For this review, take the finished solid that the model builds, in its own axes (mm). Face numbers are marked on the shaded views. A direction names the side the tool comes from. Coordinates: 2 decimals unless noted, no trailing zeros. Write each loop counter-clockwise with the first axis right and the second up, starting at its lowest first coordinate (ties: lowest second). Pieces come first, ordered by that corner, then holes. Notation, with made-up numbers: (-5, 50) -> (42, 50) arc R25 ccw to (42, 74) -> close; hole circle Ø8 at (-6.5, -5). An arc over 180 degrees is marked (long way). Put each result on its own line as item: value. Start each with the question number.
Item 1: To check wall thickness, follow L1, parallel to Z at x = -6.5, y = 19.5; L2, parallel to Z at x = 1.5, y = 15; L3, parallel to X at y = 19.25, z = -19.5. State the ranges of each line that lie inside material, in increasing order.
Item 2: Consider section A-A on y = 22. Give the number of separate pieces and of enclosed holes in the cut face, and give its area (3 significant figures).
Item 3: Consider section D-D on x = 8.5. Give the boundary of the cut face in (y, z).
Item 4: Consider section C-C on z = 9. Give the boundary of the cut face in (x, y), and give its area (3 significant figures).
Item 5: Consider section B-B on x = -12. Give the boundary of the cut face in (y, z).
Item 6: Insertion check: P1, Ø8, axis at y = 16.5, z = 10.5, coming from the -X side; P2, Ø4, axis at x = 20, y = 17, coming from the +Z side; P3, Ø1.5, axis at x = 18.5, z = 9, coming from the +Y side. Each pin has a flat end and moves straight along its axis. Give the tip position at first contact, or say it passes through.
Item 7: For the marked faces 1, 2 and 3, list the 3-axis set-ups (+Z, -Z, +X, -X, +Y, -Y) from which the entire face can be reached by the end or side of a thin tool; tool diameter is ignored.
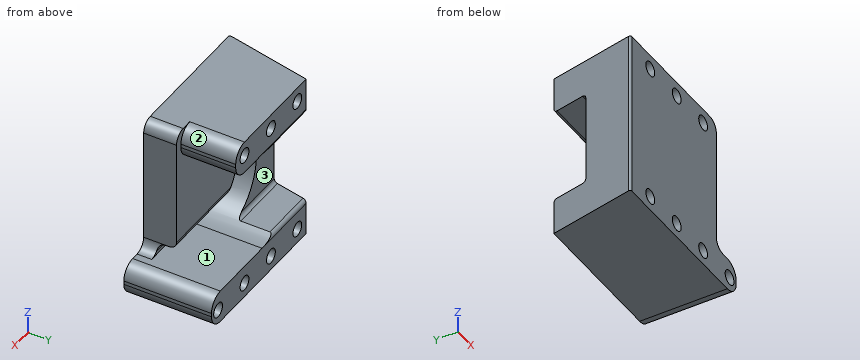
```python
from build123d import *

# Parameters (mm, degrees)
SKETCH2_R           = 2
SKETCH2_R_2         = 2.0000000000000004
SKETCH2_R_3         = 2.0000000000000036
BOSS_EXTRUDE1_DEPTH = 24
BOSS_EXTRUDE2_DEPTH = 46
CUT_EXTRUDE1_START  = -10
CUT_EXTRUDE1_DEPTH  = 10
FILLET1_R           = 1
FILLET2_R           = 0.5
FILLET3_R           = 4
BOSS_EXTRUDE3_START = -9
BOSS_EXTRUDE3_DEPTH = 9
FILLET4_R           = 3
CUT_EXTRUDE2_START  = -5
CUT_EXTRUDE2_DEPTH  = 5
FILLET5_R           = 2


with BuildPart() as part:
    # Sketch2 → Boss-Extrude1 (new body)
    with BuildSketch(Plane(origin=(0, 0, 0), x_dir=(1, 0, 0), z_dir=(0, 1, 0))):
        with BuildLine():
            ThreePointArc((-10.00000000000001, 1.71e-15), (-7.224972160321737, 8.36660026534089), (3.0642e-13, 13.41640786499884))
            ThreePointArc((3.0642e-13, 13.41640786499884), (1.9788258499060016, 13.85333371629342), (4.000000000000001, 14.00000000000001))
            Line((4, 14.00000000000001), (27, 14))
            Line((27, 14), (27, 23.000000000000007))
            Line((27, 23.000000000000007), (-16, 23))
            Line((-16, 23.000000000000004), (-16, -22.999999999999996))
            Line((-16, -22.999999999999996), (15.999999999999996, -22.999999999999993))
            Line((15.999999999999996, -22.999999999999993), (15.999999999999996, -14))
            Line((15.999999999999996, -14), (4, -14.00000000000001))
            ThreePointArc((3.9999999999999973, -14.00000000000001), (-5.899494936611674, -9.899494936611672), (-10.00000000000001, 1.71e-15))
        make_face()
        with Locations(Location((-11.999999999999995, -19, 0), (0, 0, 270))):
            Circle(SKETCH2_R, mode=Mode.SUBTRACT)
        with Locations(Location((4.65e-15, -19, 0), (0, 0, 270))):
            Circle(SKETCH2_R_2, mode=Mode.SUBTRACT)
        with Locations(Location((11.999999999999995, -19, 0), (0, 0, 270))):
            Circle(SKETCH2_R, mode=Mode.SUBTRACT)
        with Locations(Location((-12, 19, 0), (0, 0, 270))):
            Circle(SKETCH2_R_2, mode=Mode.SUBTRACT)
        with Locations(Location((4.7e-16, 19, 0), (0, 0, 270))):
            Circle(SKETCH2_R, mode=Mode.SUBTRACT)
        with Locations(Location((12, 19, 0), (0, 0, 270))):
            Circle(SKETCH2_R, mode=Mode.SUBTRACT)
        with Locations(Location((24.003693078979538, 19, 0), (0, 0, 270))):
            Circle(SKETCH2_R_3, mode=Mode.SUBTRACT)
    extrude(amount=BOSS_EXTRUDE1_DEPTH)

    # Sketch4 → Boss-Extrude2 (add)
    with BuildSketch(Plane.XY.offset(22.999999999999993)):
        Polygon((-21.000000000000004, -1.04e-15), (-16.000000000000004, 24), (-16.000000000000004, 0), align=None)
    extrude(amount=-BOSS_EXTRUDE2_DEPTH)

    # Sketch5 → Cut-Extrude1 (cut)
    with BuildSketch(Plane(origin=(0, 24, 0), x_dir=(1, 0, 0), z_dir=(0, 1, 0)).offset(CUT_EXTRUDE1_START)):
        with BuildLine():
            Line((-16, 0), (-10.000000000000007, 0))
            ThreePointArc((-10.000000000000007, 3.5391e-13), (-7.591939740998584, 7.850282354225094), (-1.1961524227063602, 13.000000000000117))
            Line((-1.196152422706339, 13), (-16, 12.999999999999998))
            Line((-16, 13.000000000000004), (-16, 0))
        make_face()
        Polygon((-21.000000000000004, 0), (-16, 0), (-16, 13.000000000000004), (-21.000000000000004, 12.999999999999998), align=None)
        with BuildLine():
            ThreePointArc((-1.1961524227063673, -13.000000000000114), (-7.591939740998785, -7.850282354224801), (-10.000000000000007, 3.5391e-13))
            Line((-10.000000000000007, 0), (-16, 0))
            Line((-16, 0), (-16, -13))
            Line((-15.999999999999998, -13.000000000000002), (-1.1961524227063371, -13))
        make_face()
        Polygon((-16, -13), (-16, 0), (-21.000000000000004, 0), (-21, -13), align=None)
    extrude(amount=CUT_EXTRUDE1_DEPTH, mode=Mode.SUBTRACT)

    # Fillet1
    fillet1_edges = [part.edges().sort_by_distance(p)[0] for p in [
        (-9.639742878019842, 14, -13.000000000000032),
        (-8.598076211353176, 24, 13.000000000000036),
        (-9.639742878019844, 14, 13.000000000000032),
        (-8.598076211353174, 24, -13.000000000000036),
    ]]
    fillet(fillet1_edges, radius=FILLET1_R - 0.0001)  # a hair under: the kernel refuses the full size

    # Fillet2
    fillet2_edges = [part.edges().sort_by_distance(p)[0] for p in [
        (-21, -1.04e-15, -7.11e-15),
    ]]
    fillet(fillet2_edges, radius=FILLET2_R)

    # Fillet3
    fillet3_edges = [part.edges().sort_by_distance(p)[0] for p in [
        (15.999999999999996, 12, 14),
        (15.999999999999996, 12, 22.999999999999993),
        (27, 12, -23.000000000000007),
        (27, 12, -14),
    ]]
    fillet(fillet3_edges, radius=FILLET3_R)

    # Sketch6 → Boss-Extrude3 (add)
    with BuildSketch(Plane.XZ.offset(BOSS_EXTRUDE3_START)):
        with BuildLine():
            ThreePointArc((4, 14.00000000000001), (-10.00000000000001, 8.6e-16), (3.9999999999999982, -14.00000000000001))
            Line((3.9999999999999964, -14.00000000000001), (18.00000000000001, -13.999999999999998))
            Line((18.00000000000001, -14.000000000000004), (18.00000000000001, 22.999999999999996))
            Line((18.00000000000001, 22.999999999999993), (11.999999999999996, 22.999999999999993))
            ThreePointArc((11.999999999999996, 22.999999999999993), (14.828427124746188, 21.828427124746185), (15.999999999999998, 18.999999999999993))
            Line((15.999999999999996, 18.999999999999993), (15.999999999999996, 18.000000000000007))
            ThreePointArc((15.999999999999996, 18.000000000000007), (14.828427124746185, 15.171572875253815), (11.999999999999993, 14.000000000000005))
            Line((11.999999999999993, 14.000000000000007), (4, 14.000000000000009))
        make_face()
    extrude(amount=BOSS_EXTRUDE3_DEPTH)

    # Fillet4
    fillet4_edges = [part.edges().sort_by_distance(p)[0] for p in [
        (18.00000000000001, 4.5, 22.999999999999993),
        (18.00000000000001, 4.5, -14),
    ]]
    fillet(fillet4_edges, radius=FILLET4_R)

    # Sketch7 → Cut-Extrude2 (cut)
    with BuildSketch(Plane(origin=(0, 9, 0), x_dir=(1, 0, 0), z_dir=(0, 1, 0)).offset(CUT_EXTRUDE2_START)):
        with BuildLine():
            Line((-4.66025403784441, 10.999999999999995), (18.00000000000001, 10.999999999999995))
            ThreePointArc((18.00000000000001, 10.999999999999995), (18.878679656440365, 13.121320343559638), (21.00000000000001, 13.999999999999995))
            Line((21.00000000000001, 13.999999999999995), (4, 14.00000000000001))
            ThreePointArc((4, 14.000000000000009), (-0.5825756949558523, 13.228756555322958), (-4.660254037844406, 10.999999999999995))
        make_face()
    extrude(amount=CUT_EXTRUDE2_DEPTH, mode=Mode.SUBTRACT)

    # Fillet5
    fillet5_edges = [part.edges().sort_by_distance(p)[0] for p in [
        (6.6698729810778, 9, -10.999999999999995),
        (6.6698729810778, 4, -10.999999999999995),
    ]]
    fillet(fillet5_edges, radius=FILLET5_R)


solid = part.part
```
Return value:
1. L1: -23 to -13, 13 to 23
1. L2: -23 to -20.32, -17.68 to -13.77, 13.77 to 17.68, 20.32 to 23
1. L3: -16.99 to -13.94, -10.06 to -1.94, 1.94 to 10.06, 13.94 to 22.07, 25.94 to 26.97
2. separate pieces: 2
2. enclosed holes: 7
2. area: 615 mm^2
3. outline: (0, -23) -> (24, -23) -> (24, -14) -> (4, -14) -> (4, -13) arc R2 cw to (6, -11) -> (7, -11) arc R2 ccw to (9, -9) -> (9, 14) -> (24, 14) -> (24, 23) -> (0, 23) -> close
4. outline: (-20.87, 0.6) arc R0.5 ccw to (-20.39, 0) -> (18, 0) -> (18, 9) -> (-6.72, 9) -> (-6.72, 14) -> (-18.08, 14) -> close
4. area: 402 mm^2
5. outline: (0, -23) -> (24, -23) -> (24, -21) -> (0, -21) -> close; (0, -17) -> (24, -17) -> (24, -14) arc R1 ccw to (23, -13) -> (15, -13) arc R1 cw to (14, -12) -> (14, 12) arc R1 cw to (15, 13) -> (23, 13) arc R1 ccw to (24, 14) -> (24, 17) -> (0, 17) -> close; (0, 21) -> (24, 21) -> (24, 23) -> (0, 23) -> close
6. P1: x = -18.4
6. P2: z = -14
6. P3: y = 9
7. face 1: +X, +Y
7. face 2: +Z, +X, +Y
7. face 3: +X, -X, +Y
